```python
from build123d import *

# Parameters (mm, degrees)
CROQUIS1_W                                           = 38
CROQUIS1_H                                           = 150
SALIENTE_EXTRUIR1_DEPTH                              = 3.175
CROQUIS3_R                                           = 6.35
CROQUIS3_R_2                                         = 1.5
CORTAR_EXTRUIR2_DEPTH                                = 25.4
AVELLANADO_PARA_TORNILLO_CON_CABEZA_OVAL_D           = 5.7912
AVELLANADO_PARA_TORNILLO_CON_CABEZA_OVAL_DEPTH       = 20
AVELLANADO_PARA_TORNILLO_CON_CABEZA_OVAL_CSINK_D     = 11.1252
AVELLANADO_PARA_TORNILLO_CON_CABEZA_OVAL_CSINK_ANGLE = 82
AVELLANADO_PARA_TORNILLO_CON_CABEZA_OVAL_TIP         = 1.739852008
CROQUIS7_R                                           = 1.984375
CORTAR_EXTRUIR3_DEPTH                                = 25.4


with BuildPart() as part:
    # Croquis1 → Saliente-Extruir1 (new, symmetric)
    with BuildSketch(Plane.XY):
        Rectangle(CROQUIS1_W, CROQUIS1_H)
    extrude(amount=SALIENTE_EXTRUIR1_DEPTH, both=True)

    # Croquis3 → Cortar-Extruir2 (cut)
    with BuildSketch(Plane.XY.offset(3.175)):
        with Locations((0, -23)):
            Circle(CROQUIS3_R)
        with Locations((-15.5, -23)):
            Circle(CROQUIS3_R_2)
        with Locations((-7.75, -9.576606241)):
            Circle(CROQUIS3_R_2)
        with Locations((7.75, -9.576606241)):
            Circle(CROQUIS3_R_2)
        with Locations((15.5, -23)):
            Circle(CROQUIS3_R_2)
        with Locations((7.75, -36.423393759)):
            Circle(CROQUIS3_R_2)
        with Locations((-7.75, -36.423393759)):
            Circle(CROQUIS3_R_2)
    extrude(amount=-CORTAR_EXTRUIR2_DEPTH, mode=Mode.SUBTRACT)

    # Avellanado para tornillo con cabeza ovalada de #121
    with Locations(Plane(origin=(-9.5, -70, 3.175), x_dir=(1, 0, 0), z_dir=(0, 0, 1))):
        with Locations((0, 0), (19, 0)):
            CounterSinkHole(AVELLANADO_PARA_TORNILLO_CON_CABEZA_OVAL_D / 2, AVELLANADO_PARA_TORNILLO_CON_CABEZA_OVAL_CSINK_D / 2, depth=AVELLANADO_PARA_TORNILLO_CON_CABEZA_OVAL_DEPTH, counter_sink_angle=AVELLANADO_PARA_TORNILLO_CON_CABEZA_OVAL_CSINK_ANGLE)
            with Locations((0, 0, -(AVELLANADO_PARA_TORNILLO_CON_CABEZA_OVAL_DEPTH + AVELLANADO_PARA_TORNILLO_CON_CABEZA_OVAL_TIP / 2))):  # 118° drill point
                Cone(0, AVELLANADO_PARA_TORNILLO_CON_CABEZA_OVAL_D / 2, AVELLANADO_PARA_TORNILLO_CON_CABEZA_OVAL_TIP, mode=Mode.SUBTRACT)

    # Croquis7 → Cortar-Extruir3 (cut)
    with BuildSketch(Plane.XY.offset(3.175)):
        with Locations((9.5, 68)):
            Circle(CROQUIS7_R)
        with Locations((-9.5, 68)):
            Circle(CROQUIS7_R)
    extrude(amount=-CORTAR_EXTRUIR3_DEPTH, mode=Mode.SUBTRACT)


solid = part.part
```
The listing builds one solid part. Answer for the finished solid, in the listing's coordinates (mm). Coordinates: 2 decimals unless noted, no trailing zeros. Loops run counter-clockwise (first coordinate to the right, second up) from the corner with the lowest first, then second, coordinate; pieces in that order, holes last. Notation, with made-up numbers: (17.5, -31) -> (73.5, -31) arc R19 ccw to (73.5, -27) -> close; hole circle Ø3 at (81, 56.25). An arc over 180 degrees is marked (long way). Return JSON: item names as keys, results as strings. Group by question number.
(1) A cutting plane is placed at C-C on z = -1.75. Count the separate pieces of the cut face and the enclosed holes in it, and give its area (3 significant figures).
(2) Find the intervals of material crossed by probe 1 along Y at (x, z) = (-9.5, -0.5); probe 2 along X at (y, z) = (-70, -2.4); probe 3 along Y at (x, z) = (0, 1.75), in increasing order. Write a range as from..to.
(3) Determine the mould class of faces 1 (the flat face through (0, 75, 0)), 2 (the cylindrical face through (9.88, -67.13, -1.56)), 3 (the flat face through (19, -1, 0)) for opening direction Y: released by +Y, released by -Y, zero draft, split by the parting line, or undercut.
(4) A cutting plane is placed at B-B on x = 0. Write down the section's boundary in (y, z) (3 decimals), and give its area (3 significant figures).
(5) A cutting plane is placed at A-A on y = -23. Write down the section's boundary in (x, z) (3 decimals), and give its area (3 significant figures).
The answers:
{
 "1": {"separate pieces": "1", "enclosed holes": "11", "area": "5,450 mm^2"},
 "2": {"probe 1": "y = -75..-72.9, -67.1..66.02, 69.98..75", "probe 2": "x = -19..-12.4, -6.6..6.6, 12.4..19", "probe 3": "y = -75..-29.35, -16.65..75"},
 "3": {"face 1": "released by +Y", "face 2": "undercut", "face 3": "zero draft"},
 "4": {"outline": "(-75, -3.175) -> (-29.35, -3.175) -> (-29.35, 3.175) -> (-75, 3.175) -> close; (-16.65, -3.175) -> (75, -3.175) -> (75, 3.175) -> (-16.65, 3.175) -> close", "area": "872 mm^2"},
 "5": {"outline": "(-19, -3.175) -> (-17, -3.175) -> (-17, 3.175) -> (-19, 3.175) -> close; (-14, -3.175) -> (-6.35, -3.175) -> (-6.35, 3.175) -> (-14, 3.175) -> close; (6.35, -3.175) -> (14, -3.175) -> (14, 3.175) -> (6.35, 3.175) -> close; (17, -3.175) -> (19, -3.175) -> (19, 3.175) -> (17, 3.175) -> close", "area": "123 mm^2"}
}
